Work out the finished part from the listing and answer in its coordinate system (mm). A direction names the side the tool comes from. Coordinates: 2 decimals unless noted, no trailing zeros. Write each loop counter-clockwise with the first axis right and the second up, starting at its lowest first coordinate (ties: lowest second). Pieces come first, ordered by that corner, then holes. Notation, with made-up numbers: (-12.75, -19.75) - (22.25, -19.75) arc R23 ccw to (22.25, -8.75) - close; hole circle Ø4 at (-31, -2.75). An arc over 180 degrees is marked (long way). Use one line per item in the form item = value. Start each with the question number.
Item 1: Given pin 1 (1.8 mm diameter, centred on x = -0.5, y = 3.5, fed in from -Z); pin 2 (1.2 mm diameter, centred on x = -1, z = 2.5, fed in from +Y); pin 3 (1.5 mm diameter, centred on y = -2, z = 14, fed in from -X), each flat-ended and moving along its own axis, determine where each tip first touches the part or whether it passes through.
Item 2: Consider probe 1 along Z at (x, y) = (-3, -1.75); probe 2 along Y at (x, z) = (-2.5, 3.5); probe 3 along Z at (x, y) = (3, -2.25). Determine where each line is inside the solid, lowest interval first.
Item 3: A cutting plane is placed at A-A (x = 0). Write down the section's boundary in (y, z).
Item 4: Determine the mould class of faces 1 (the flat face through (0, -3, 4)), 2 (the flat face through (0, 0, 38)), 3 (the flat face through (1, 3, 19)) for opening direction Z: released by +Z, released by -Z, zero draft, split by the parting line, or undercut.
Item 5: For faces 4 (the conical face through (3.64, -0.04, 0.14)), 5 (the flat face through (0, -2.331, 2)), 6 (the flat face through (1, 3, 18)), 7 (the flat face through (0, 3, 4)), determine the directions among +Z, -Z, +X, -X, +Y, -Y from which every point of the face is accessible in a straight line to the end or side of a thin tool.
Item 6: A cutting plane is placed at B-B (z = 31). Write down the section's boundary in (x, y), then the cut area to 3 significant figures.
from build123d import *

# Parameters (mm, degrees)
ESQUISSE1_R             = 4
BASE_EXTRUSION_DEPTH    = 38
CHANFREIN1_SIZE         = 0.5
ESQUISSE2_OUTSIDE_W     = 17.93
ESQUISSE2_OUTSIDE_H     = 17.93
ESQUISSE2_OUTSIDE_R     = 3
ENL_V_MAT_EXTRU_1_DEPTH = 1
ESQUISSE3_OUTSIDE_W     = 17.93
ESQUISSE3_OUTSIDE_H     = 17.93
ENL_V_MAT_EXTRU_2_DEPTH = 4


with BuildPart() as part:
    # Esquisse1 → Base-Extrusion (new body)
    with BuildSketch(Plane.XY):
        with Locations(Location((0, 0, 0), (0, 0, 215.635694855))):
            Circle(ESQUISSE1_R)
    extrude(amount=BASE_EXTRUSION_DEPTH)

    # Chanfrein1
    chanfrein1_edges = [part.edges().sort_by_distance(p)[0] for p in [
        (3.25095178, 2.330517652, 0),
        (3.25095178, 2.330517652, 38),
    ]]
    chamfer(chanfrein1_edges, length=CHANFREIN1_SIZE)

    # Esquisse2 outside → Enlèv. mat.-Extru.1 (cut)
    with BuildSketch(Plane.XY.offset(19)):
        Rectangle(ESQUISSE2_OUTSIDE_W, ESQUISSE2_OUTSIDE_H)
        Circle(ESQUISSE2_OUTSIDE_R, mode=Mode.SUBTRACT)
    extrude(amount=-ENL_V_MAT_EXTRU_1_DEPTH, mode=Mode.SUBTRACT)

    # Esquisse3 outside → Enlèv. mat.-Extru.2 (cut)
    with BuildSketch(Plane(origin=(0, 0, 0), x_dir=(-1, 0, 0), z_dir=(0, 0, -1))):
        Rectangle(ESQUISSE3_OUTSIDE_W, ESQUISSE3_OUTSIDE_H)
        with BuildLine():
            Line((-3.25095178, 2.330517652), (3.25095178, 2.330517652))
            ThreePointArc((3.25095178, 2.330517652), (4, 0), (3.25095178, -2.330517652))
            Line((3.25095178, -2.330517652), (-3.25095178, -2.330517652))
            ThreePointArc((-3.25095178, -2.330517652), (-4, 0), (-3.25095178, 2.330517652))
        make_face(mode=Mode.SUBTRACT)
    extrude(amount=-ENL_V_MAT_EXTRU_2_DEPTH, mode=Mode.SUBTRACT)


solid = part.part
Answer:
q1.pin_1 = 4
q1.pin_2 = 2.33
q1.pin_3 = -3.8
q2.probe_1 = 0 to 18, 19 to 38
q2.probe_2 = -2.33 to 2.33
q2.probe_3 = 0.25 to 18, 19 to 37.75
q3.outline = (-4, 4) - (-2.33, 4) - (-2.33, 0) - (2.33, 0) - (2.33, 4) - (4, 4) - (4, 18) - (3, 18) - (3, 19) - (4, 19) - (4, 37.5) - (3.5, 38) - (-3.5, 38) - (-4, 37.5) - (-4, 19) - (-3, 19) - (-3, 18) - (-4, 18) - close
q4.face_1 = released by -Z
q4.face_2 = released by +Z
q4.face_3 = undercut
q5.face_4 = -Z, +X
q5.face_5 = -Z, +X, -X, -Y
q5.face_6 = none
q5.face_7 = -Z, +X, -X, +Y
q6.outline = circle Ø8 at (0, 0)
q6.area = 50.3 mm²
